Geometry check sheet. Reference: the model listing, model coordinates, mm. Round coordinates to 2 decimals unless told otherwise and drop trailing zeros. Order: outer loops, then holes, each group sorted by start corner. A loop starts at its lowest first (then second) coordinate and runs counter-clockwise, first axis right, second up.
(1) Cross-section at C-C on y = -1.75. Enter the section's corners in (x, z), and give its area (3 significant figures).
(2) Cross-section at A-A on x = 0. Enter the section's corners in (y, z).
(3) Thickness scan on L1, parallel to Z at x = 0, y = 5; L2, parallel to X at y = 2.5, z = -164.5. Record the ranges inside material, lowest first.
(4) Cross-section at B-B on z = -119. Enter the section's corners in (x, y).
(5) Gauge pin test, flat ends, axial feed: P1, Ø0.5, axis at y = 4, z = -238.5, coming from the +X side; P2, Ø0.8, axis at y = 4.5, z = 0.5, coming from the +X side; P3, Ø4.5, axis at x = 0, z = 0.5, coming from the +Y side. Record the tip position at first contact, or that the pin passes through.
from build123d import *

# Parameters (mm, degrees)
SKETCH_1_R          = 5.5
EXTRUDE_1_DEPTH     = 275
CUT_EXTRUDE_1_DEPTH = 2
CUT_EXTRUDE_2_DEPTH = 2
CUT_EXTRUDE_3_DEPTH = 2


with BuildPart() as part:
    # 草图1 → 凸台-拉伸1 (new, symmetric)
    with BuildSketch(Plane.XY):
        Circle(SKETCH_1_R)
    extrude(amount=EXTRUDE_1_DEPTH, both=True)

    # 草图2 → 切除-拉伸1 (cut)
    with BuildSketch(Plane(origin=(0, 5.5, 0), x_dir=(1, 0, 0), z_dir=(0, 1, 0))):
        with BuildLine():
            Line((2, 3), (2, -3))
            ThreePointArc((2, -3), (0, -5), (-2, -3))
            Line((-2, -3), (-2, 3))
            ThreePointArc((-2, 3), (0, 5), (2, 3))
        make_face()
    extrude(amount=-CUT_EXTRUDE_1_DEPTH, mode=Mode.SUBTRACT)

    # 草图3 → 切除-拉伸2 (cut)
    with BuildSketch(Plane(origin=(0, 5.5, 0), x_dir=(1, 0, 0), z_dir=(0, 1, 0))):
        with BuildLine():
            Line((2, 173), (2, 167))
            ThreePointArc((2, 167), (0, 165), (-2, 167))
            Line((-2, 167), (-2, 173))
            ThreePointArc((-2, 173), (0, 175), (2, 173))
        make_face()
        with BuildLine():
            Line((2, -173), (2, -167))
            ThreePointArc((2, -167), (0, -165), (-2, -167))
            Line((-2, -167), (-2, -173))
            ThreePointArc((-2, -173), (0, -175), (2, -173))
        make_face()
    extrude(amount=-CUT_EXTRUDE_2_DEPTH, mode=Mode.SUBTRACT)

    # 草图4 → 切除-拉伸3 (cut)
    with BuildSketch(Plane(origin=(0, 5.5, 0), x_dir=(1, 0, 0), z_dir=(0, 1, 0))):
        with BuildLine():
            Line((-2, -242.77797753), (-2, -227.77797753))
            ThreePointArc((-2, -227.77797753), (0, -225.77797753), (2, -227.77797753))
            Line((2, -227.77797753), (2, -242.77797753))
            ThreePointArc((2, -242.77797753), (0, -244.77797753), (-2, -242.77797753))
        make_face()
        with BuildLine():
            Line((-2, 242.77797753), (-2, 227.77797753))
            ThreePointArc((-2, 227.77797753), (0, 225.77797753), (2, 227.77797753))
            Line((2, 227.77797753), (2, 242.77797753))
            ThreePointArc((2, 242.77797753), (0, 244.77797753), (-2, 242.77797753))
        make_face()
    extrude(amount=-CUT_EXTRUDE_3_DEPTH, mode=Mode.SUBTRACT)


solid = part.part
Found:
1. outline: (-5.21, -275) - (5.21, -275) - (5.21, 275) - (-5.21, 275) - close
1. area: 5,740 mm2
2. outline: (-5.5, -275) - (5.5, -275) - (5.5, -244.78) - (3.5, -244.78) - (3.5, -225.78) - (5.5, -225.78) - (5.5, -175) - (3.5, -175) - (3.5, -165) - (5.5, -165) - (5.5, -5) - (3.5, -5) - (3.5, 5) - (5.5, 5) - (5.5, 165) - (3.5, 165) - (3.5, 175) - (5.5, 175) - (5.5, 225.78) - (3.5, 225.78) - (3.5, 244.78) - (5.5, 244.78) - (5.5, 275) - (-5.5, 275) - close
3. L1: z = -275 to -244.78, -225.78 to -175, -165 to -5, 5 to 165, 175 to 225.78, 244.78 to 275
3. L2: x = -4.9 to 4.9
4. outline: circle Ø11 at (0, 0)
5. P1: stops at x = 4.02
5. P2: stops at x = 3.67
5. P3: stops at y = 5.12
